CAD build for the part. Positions are in the model's coordinates, mm. A direction names the side the tool comes from. Round coordinates to 2 decimals unless told otherwise and drop trailing zeros. Loops run counter-clockwise (first coordinate to the right, second up) from the corner with the lowest first, then second, coordinate; pieces in that order, holes last. Notation, with made-up numbers: M 75,-13.75 L 118,-13.75 A18 ccw 118,5.25 Z; hole C 36.5,83.25 d3. An arc over 180 degrees is marked long. Put each result on its own line as item: value. Start each with the question number.
from build123d import *

# Parameters (mm, degrees)
BOSS_EXTRUDE1_DEPTH = 16
SKETCH2_W           = 10
SKETCH2_H           = 18.7
BOSS_EXTRUDE2_DEPTH = 3
CUT_EXTRUDE1_REACH  = 33.7
SKETCH3_R           = 0.5


with BuildPart() as part:
    # Sketch1 → Boss-Extrude1 (new body)
    with BuildSketch(Plane(origin=(0, 0, 0), x_dir=(0, 0, -1), z_dir=(1, 0, 0))):
        Polygon((25, 0), (0, 0), (0, 31.7), (5.035, 31.7), (13, 31.7), (13, 21.7), (3, 21.7), (3, 16.7), (5.4, 16.7), (5.4, 13), (3, 13), (3, 3), (25, 3), align=None)
    extrude(amount=BOSS_EXTRUDE1_DEPTH)

    # Sketch2 → Boss-Extrude2 (add)
    with BuildSketch(Plane(origin=(16, 0, 0), x_dir=(0, 0, -1), z_dir=(1, 0, 0))):
        with Locations((8, 12.35)):
            Rectangle(SKETCH2_W, SKETCH2_H)
    extrude(amount=-BOSS_EXTRUDE2_DEPTH)

    # Sketch3 → Cut-Extrude1 (cut, up to next)
    with BuildSketch(Plane(origin=(0, 31.7, 0), x_dir=(1, 0, 0), z_dir=(0, 1, 0)), mode=Mode.PRIVATE) as cut_extrude1_sk1:
        with Locations((6.75, 4.5)):
            Circle(SKETCH3_R)
    cut_extrude1_tool1 = extrude(cut_extrude1_sk1.sketch, amount=-CUT_EXTRUDE1_REACH, mode=Mode.PRIVATE) & part.part
    add(cut_extrude1_tool1.solids().sort_by_distance((6.75, 31.7, -4.5))[0], mode=Mode.SUBTRACT)


solid = part.part
(1) Drill centre lines: line 1 along X through (y, z) = (26.75, -4.5); line 2 along Y through (x, z) = (10, -4.75); line 3 along Z through (x, y) = (6.75, 29). Where is each one in solid material? Low to high.
(2) Tool access for faces 1 (the flat face through (8, 3, -14)), 2 (the flat face through (8, 31.7, -7)), 3 (the cylindrical face through (7.02, 26.77, -4.92)): list every direction of +Z, -Z, +X, -X, +Y, -Y with a clear straight run to the whole face (end or side of a thin tool).
(3) Cut at B-B on x = 6.75. List the corners of the cut face in (y, z), and give its area (3 significant figures).
(4) Mould opens along Y. For faces 4 (the flat face through (8, 0, -13)), 5 (the flat face through (6, 15, -5.4)), 6 (the flat face through (13, 12, -8)), 7 (the flat face through (10, 24, -13)) say: +Y half, -Y half, draft (parallel to the pull), parting line (faces both ways), or undercut.
(5) Flat gauge pins, fed straight in: pin 1 Ø4 at (x, y) = (9, 13.5) entering from -Z; pin 2 Ø12 at (y, z) = (23, -20) entering from -X; pin 3 Ø6 at (x, y) = (13.5, 20) entering from -Z; pin 4 Ø2.5 at (x, y) = (5.5, 18) entering from -Z. Where does each tip first touch, or does it go through?
(6) Cut at C-C on y = 26.5. List the corners of the cut face in (x, z).
(7) Cut at A-A on z = -4.5. List the corners of the cut face in (x, y), and give its area (3 significant figures).
(8) Cut at D-D on y = 19.5. List the corners of the cut face in (x, z), and give its area (3 significant figures).
Taken from the geometry:
1. line 1: 0 to 6.25, 7.25 to 16
1. line 2: 0 to 3, 13 to 16.7, 21.7 to 31.7
1. line 3: -13 to -5, -4 to 0
2. face 1: -Z, -X
2. face 2: +Z, -Z, +X, -X, +Y
2. face 3: +Y
3. outline: M 0,-25 L 3,-25 L 3,-3 L 13,-3 L 13,-5.4 L 16.7,-5.4 L 16.7,-3 L 21.7,-3 L 21.7,-4 L 31.7,-4 L 31.7,0 L 0,0 Z; M 21.7,-13 L 31.7,-13 L 31.7,-5 L 21.7,-5 Z
3. area: 260 mm2
4. face 4: -Y half
4. face 5: undercut
4. face 6: undercut
4. face 7: draft
5. pin 1: z = -5.4
5. pin 2: through
5. pin 3: z = -13
5. pin 4: z = -3
6. outline: M 0,-13 L 16,-13 L 16,0 L 0,0 Z; hole C 6.75,-4.5 d1
7. outline: M 0,0 L 16,0 L 16,31.7 L 7.25,31.7 L 7.25,21.7 L 13,21.7 L 13,16.7 L 0,16.7 L 0,13 L 13,13 L 13,3 L 0,3 Z; M 0,21.7 L 6.25,21.7 L 6.25,31.7 L 0,31.7 Z
7. area: 302 mm2
8. outline: M 0,-3 L 13,-3 L 13,-13 L 16,-13 L 16,0 L 0,0 Z
8. area: 78.0 mm2
